from build123d import *

# Parameters (mm, degrees)
F1_DEPTH = 10
F2_W     = 4
F2_H     = 4
F3_DEPTH = 4
F4_SIZE  = 1


with BuildPart() as f1:
    # F0 (on Top) → F1 (new body)
    with BuildSketch(Plane.XY):
        Polygon((0, 11), (0, 0), (6.5, 11.2583302492), (6.5, 40.2583302492), (-18.9234679854, -9.6380351054), (-9.72022002, -9.8450791018), align=None)
    extrude(amount=F1_DEPTH)

    # F2 (on face) → F3 (join)
    with BuildSketch(Plane(origin=(-0.2262881219, -10.0586625682, 0), x_dir=(0.9997470421, -0.0224911492, 0), z_dir=(-0.0224911492, -0.9997470421, 0))):
        with Locations((-14.0991223651, 5)):
            Rectangle(F2_W, F2_H)
    extrude(amount=F3_DEPTH)

    # F4
    f4_edges = [f1.edges().sort_by_distance(p)[0] for p in [
        (-4.86011, 0.57746, 10),
        (0, 5.5, 10),
        (3.25, 5.629165, 10),
        (6.5, 25.75833, 10),
        (-6.211734, 15.310148, 10),
        (6.5, 25.75833, 0),
        (-6.211734, 15.310148, 0),
        (3.25, 5.629165, 0),
        (0, 5.5, 0),
        (-4.86011, 0.57746, 0),
    ]]
    chamfer(f4_edges, length=F4_SIZE)


solid = f1.part
Can you work these out from the model? Positions are in its coordinate system, mm. A direction names the side the tool comes from. Coordinates: 2 decimals unless noted, no trailing zeros. Write each loop counter-clockwise with the first axis right and the second up, starting at its lowest first coordinate (ties: lowest second). Pieces come first, ordered by that corner, then holes. Notation, with made-up numbers: (0, 58) - (6, 58) arc R21 cw to (6, 70) - close; hole circle Ø10 at (-25, 16.5). An arc over 180 degrees is marked (long way). Return JSON: item names as keys, results as strings. Group by question number.
Item 1: Please list where these lines run through material, in increasing order: probe 1 along X at (y, z) = (5.5, 1.75); probe 2 along X at (y, z) = (7, 6.5); probe 3 along X at (y, z) = (-10, 3.25).
Item 2: If we section it at D-D (y = 31): Write out the boundary of the cut face in (x, z), then the cut area to 3 significant figures.
Item 3: If we section it at A-A (z = 6.5): Write out the boundary of the cut face in (x, y), then the cut area to 3 significant figures.
Item 4: We'd pull the mould along X, two halves only. Please class faces 1 (the face through (3.205, 5.55, 4.944)), 2 (the face through (0.5, 7.9, 0.5)), 3 (the face through (-5.595, 15.436, 9.493)): pulls with the +X half, pulls with the -X half, needs draft (parallel to the pull), parting line crosses it, or undercut.
Item 5: Which directions (+Z, -Z, +X, -X, +Y, -Y) give clear straight access to the entire face, cutting with the end or side of a thin tool? Please do faces 4 (the face through (-4.542, 2.459, 0.493)), 5 (the face through (-4.93, 0.43, 4.94)), 6 (the face through (6.5, 26, 5)), 7 (the face through (-4.542, 2.459, 9.507)), 8 (the face through (6, 25.6, 0.5)).
Item 6: I'm going to push flat-ended pins straight in: pin 1 Ø2 at (x, y) = (-14.5, -11.5) entering from -Z; pin 2 Ø4.5 at (x, y) = (-15, -11.5) entering from +Z; pin 3 Ø2 at (y, z) = (-5.5, 4.5) entering from +X; pin 4 Ø4 at (y, z) = (7.5, 5) entering from +X. Where does each tip first touch, or does it pass through?
Item 7: If we section it at B-B (y = 7): Write out the boundary of the cut face in (x, z).
Item 8: If we section it at C-C (x = -14.75): Write out the boundary of the cut face in (y, z).
Return value:
{
 "1": {"probe 1": "x = -11.21 to -2.56, 0 to 3.18", "probe 2": "x = -10.45 to -1.87, 0 to 4.04", "probe 3": "x = -16.33 to -12.33"},
 "2": {"outline": "(1.78, 1) - (2.9, 0) - (5.5, 0) - (6.5, 1) - (6.5, 9) - (5.5, 10) - (2.9, 10) - (1.78, 9) - close", "area": "45.1 mm^2"},
 "3": {"outline": "(-18.92, -9.64) - (-16.32, -9.7) - (-16.41, -13.7) - (-12.41, -13.79) - (-12.32, -9.79) - (-9.72, -9.85) - (0, 11) - (0, 0) - (6.5, 11.26) - (6.5, 40.26) - close", "area": "453 mm^2"},
 "4": {"face 1": "pulls with the +X half", "face 2": "undercut", "face 3": "pulls with the -X half"},
 "5": {"face 4": "-Z, -Y", "face 5": "+Z, -Z, -Y", "face 6": "+Z, -Z, +X, +Y, -Y", "face 7": "+Z, -Y", "face 8": "-Z, +X, +Y, -Y"},
 "6": {"pin 1": "stops at z = 3", "pin 2": "stops at z = 10", "pin 3": "stops at x = -7.23", "pin 4": "stops at x = 5.48"},
 "7": {"outline": "(-10.45, 1) - (-9.32, 0) - (-2.97, 0) - (-1.87, 1) - (-1.87, 9) - (-2.97, 10) - (-9.32, 10) - (-10.45, 9) - close; (0, 1) - (1, 0) - (2.89, 0) - (4.04, 1) - (4.04, 9) - (2.89, 10) - (1, 10) - (0, 9) - close"},
 "8": {"outline": "(-13.73, 3) - (-9.73, 3) - (-9.73, 0) - (-3.65, 0) - (-1.45, 1) - (-1.45, 9) - (-3.65, 10) - (-9.73, 10) - (-9.73, 7) - (-13.73, 7) - close"}
}
